Input: part model. Units: mm. Frame: model coordinates. A direction names the side the tool comes from. Round coordinates to 2 decimals unless told otherwise and drop trailing zeros. Loops run counter-clockwise (first coordinate to the right, second up) from the corner with the lowest first, then second, coordinate; pieces in that order, holes last. Notation, with made-up numbers: (35, -16) -> (44, -16) arc R38 cw to (44, 22) -> close; hole circle Ø6 at (-33.5, 49.5). An arc over 180 degrees is marked (long way). Answer in a Markdown table with one row per item. Add a question column.
Q1. Section A-A, the plane y = 19.05. Output: boundary loops of the cut face in (x, z) (1 decimal).
Q2. Section B-B, the plane z = -17.5. Output: boundary loops of the cut face in (x, y).
Q3. Mould query, pull axis X, two halves, no side actions, for faces 5 (the face through (17.738, 20.863, -40.59)), 6 (the face through (11, 6.35, -10)), 7 (the face through (27.454, 28.53, -40.59)), 8 (the face through (44.525, 3, -2)). Classes: pulls with the +X half, pulls with the -X half, needs draft (parallel to the pull), parting line crosses it, or undercut.
Q4. Pin query (flat end, axial travel): pin 1 (7 mm diameter, centred on x = -4.5, y = 2, fed in from -Z); pin 2 (5 mm diameter, centred on x = 28.44, y = 26.99, fed in from +Z) (3 decimals); pin 3 (8 mm diameter, centred on y = 12, z = -35, fed in from +X). Return the tip coordinate at first contact, or that it passes through.
Q5. Section D-D, the plane y = 26. Output: boundary loops of the cut face in (x, z) (1 decimal), and give its area (3 significant figures).
Q6. Ray query, L1, parallel to X at y = 12, z = -41; L2, parallel to Y at x = 11, z = -10.5; L3, parallel to Y at x = 32.5, z = -2. Return the intervals inside material, ascending. Write a range as from..to.
Q7. Section C-C, the plane x = 17.5. Give the number of separate pieces and of enclosed holes in the cut face, and give its area (3 significant figures).
Q8. Reachability of faces 1 (the face through (17, 22, -38.175)), 2 (the face through (15.256, 0.751, -27.604)), 3 (the face through (-5, 3, -4.762)), 4 (the face through (40, 3, -4.762)) from +Z, -Z, +X, -X, +Y, -Y: full face, straight path, thin tool, end or side. Return the list, or none.
```python
from build123d import *

# Parameters (mm, degrees)
SKETCH1_W                 = 35
SKETCH1_H                 = 42.9375
BOSS_EXTRUDE1_DEPTH       = 6.35
SKETCH2_W                 = 35
SKETCH2_H                 = 4.7625
BOSS_EXTRUDE2_DEPTH       = 25.4
SKETCH3_R                 = 8.763
CUT_EXTRUDE1_DEPTH        = 32.75
F_6_CLEARANCE_HOLE1_D     = 3.6576
SKETCH13_R                = 10.3505
SKETCH13_R_2              = 8.763
CUT_EXTRUDE2_DEPTH        = 1.524
SKETCH14_W                = 9.525
SKETCH14_H                = 4.7625
BOSS_EXTRUDE4_DEPTH       = 6.35
F_4_CLEARANCE_HOLE1_D     = 3.2639
F_4_CLEARANCE_HOLE1_DEPTH = 10.16
F_4_CLEARANCE_HOLE1_TIP   = 0.980574487


with BuildPart() as part:
    # Sketch1 → Boss-Extrude1 (new body)
    with BuildSketch(Plane(origin=(0, 0, 0), x_dir=(1, 0, 0), z_dir=(0, 1, 0))):
        with Locations((17.5, 21.46875)):
            Rectangle(SKETCH1_W, SKETCH1_H)
    extrude(amount=BOSS_EXTRUDE1_DEPTH)

    # Sketch2 → Boss-Extrude2 (add)
    with BuildSketch(Plane(origin=(0, 6.35, 0), x_dir=(1, 0, 0), z_dir=(0, 1, 0))):
        with Locations((17.5, 40.55625)):
            Rectangle(SKETCH2_W, SKETCH2_H)
    extrude(amount=BOSS_EXTRUDE2_DEPTH)

    # Sketch3 → Cut-Extrude1 (cut, through all)
    with BuildSketch(Plane.XZ):
        with Locations((17.5, -17.5)):
            Circle(SKETCH3_R)
    extrude(amount=-CUT_EXTRUDE1_DEPTH, mode=Mode.SUBTRACT)

    # #6 Clearance Hole1 (through all)
    with Locations(Plane.XY.offset(-38.175)):
        with Locations((6.5625, 26.9875), (17.5, 19.05), (6.5625, 11.1125), (28.4375, 26.9875), (28.4375, 11.1125)):
            Hole(F_6_CLEARANCE_HOLE1_D / 2)

    # Sketch13 → Cut-Extrude2 (cut)
    with BuildSketch(Plane.XZ):
        with Locations((17.5, -17.5)):
            Circle(SKETCH13_R)
        with Locations((17.5, -17.5)):
            Circle(SKETCH13_R_2, mode=Mode.SUBTRACT)
    extrude(amount=-CUT_EXTRUDE2_DEPTH, mode=Mode.SUBTRACT)

    # Sketch14 → Boss-Extrude4 (add)
    with BuildSketch(Plane.XZ):
        with Locations((39.7625, -2.38125)):
            Rectangle(SKETCH14_W, SKETCH14_H)
        with Locations((-4.7625, -2.38125)):
            Rectangle(SKETCH14_W, SKETCH14_H)
    extrude(amount=-BOSS_EXTRUDE4_DEPTH)

    # #4 Clearance Hole1
    with Locations(Plane(origin=(0, 0, 0), x_dir=(-1, 0, 0), z_dir=(0, -1, 0))):
        with Locations((4.7625, 2.38125), (-39.7625, 2.38125)):
            Hole(F_4_CLEARANCE_HOLE1_D / 2, depth=F_4_CLEARANCE_HOLE1_DEPTH)
            with Locations((0, 0, -(F_4_CLEARANCE_HOLE1_DEPTH + F_4_CLEARANCE_HOLE1_TIP / 2))):  # 118° drill point
                Cone(0, F_4_CLEARANCE_HOLE1_D / 2, F_4_CLEARANCE_HOLE1_TIP, mode=Mode.SUBTRACT)


solid = part.part
```
Answer block:
| question | item | result |
|---|---|---|
| 1 | outline | (0, -42.9) -> (15.7, -42.9) -> (15.7, -38.2) -> (0, -38.2) -> close; (19.3, -42.9) -> (35, -42.9) -> (35, -38.2) -> (19.3, -38.2) -> close |
| 2 | outline | (0, 0) -> (7.15, 0) -> (7.15, 1.52) -> (8.74, 1.52) -> (8.74, 6.35) -> (0, 6.35) -> close; (26.26, 1.52) -> (27.85, 1.52) -> (27.85, 0) -> (35, 0) -> (35, 6.35) -> (26.26, 6.35) -> close |
| 3 | face 5 | undercut |
| 3 | face 6 | needs draft |
| 3 | face 7 | undercut |
| 3 | face 8 | pulls with the +X half |
| 4 | pin 1 | z = -4.76 |
| 4 | pin 2 | z = -38.175 |
| 4 | pin 3 | x = 35 |
| 5 | outline | (0, -42.9) -> (5, -42.9) -> (5, -38.2) -> (0, -38.2) -> close; (8.1, -42.9) -> (26.9, -42.9) -> (26.9, -38.2) -> (8.1, -38.2) -> close; (30, -42.9) -> (35, -42.9) -> (35, -38.2) -> (30, -38.2) -> close |
| 5 | area | 137 mm^2 |
| 6 | L1 | 0..4.96, 8.16..26.84, 30.04..35 |
| 6 | L2 | 1.52..6.35 |
| 6 | L3 | 0..6.35 |
| 7 | separate pieces | 3 |
| 7 | enclosed holes | 0 |
| 7 | area | 260 mm^2 |
| 8 | face 1 | +Z, +X, -X, +Y |
| 8 | face 2 | -Y |
| 8 | face 3 | -Z, -X, +Y, -Y |
| 8 | face 4 | -Z, +X, +Y, -Y |
